Design review of the part built by this model. Coordinates are the model's own, in mm. Face numbers are marked on the shaded views. A direction names the side the tool comes from. Coordinates: 2 decimals unless noted, no trailing zeros. Write each loop counter-clockwise with the first axis right and the second up, starting at its lowest first coordinate (ties: lowest second). Pieces come first, ordered by that corner, then holes.
Q1. Take a section at B-B, the plane x = -13.5. Write out the cut boundary in (y, z), plus the area to 3 significant figures.
Q2. Take a section at C-C, the plane z = 41. Write out the cut boundary in (x, y), plus the area to 3 significant figures.
Q3. For the marked faces 1 and 2, list the 3-axis set-ups (+Z, -Z, +X, -X, +Y, -Y) from which the entire face can be reached by the end or side of a thin tool; tool diameter is ignored.
Q4. Take a section at A-A, the plane z = 52. Write out the cut boundary in (x, y), plus the area to 3 significant figures.
Q5. Take a section at D-D, the plane x = -29. Write out the cut boundary in (y, z).
Q6. For L1, parallel to Z at x = -37.5, y = 0.35; L2, parallel to Z at x = -13.5, y = 0.3; L3, parallel to Z at x = -11, y = 1.95, list the stretches that pass through material, from the lowest coordinate up.
Q7. For pin 1 Ø0.9 at (y, z) = (-0.5, 7.5) entering from -X; pin 2 Ø3.5 at (x, z) = (-37.5, 52) entering from +Y; pin 3 Ø0.7 at (x, y) = (-2, 0.5) entering from -Z, all flat-tipped, find the tip position at first contact; note any pin that passes through.
Autodesk Inventor part; units mm, degrees
ref_plane "YZ Plane" through (0, 0, 0) normal (1, 0, 0) x (0, 1, 0)
ref_plane "XZ Plane" through (0, 0, 0) normal (0, 1, 0) x (-1, 0, 0)
ref_plane "XY Plane" through (0, 0, 0) normal (0, 0, 1) x (1, 0, 0)
sketch "Sketch1" plane through (0, 0, 0) normal (0, 1, 0) x (-1, 0, 0)
  line L0 (40, 70) -> (0, 70)
  line L1 (0, 70) -> (0, 0)
  line L2 (0, 0) -> (40, 0)
  line L3 (40, 0) -> (40, 70)
  line L4 (0, 4) -> (7.5, 4)
  line L5 (7.5, 4) -> (7.5, 0)
  line L6 (7.5, 0) -> (0, 0)
  line L7 (0, 0) -> (0, 4)
  line L8 (0, 70) -> (7.5, 70)
  line L9 (7.5, 70) -> (7.5, 66)
  line L10 (7.5, 66) -> (0, 66)
  line L11 (0, 66) -> (0, 70)
  line L12 (0, 11) -> (3.0528, 11)
  line L13 (3.5, 11.4472) -> (3.5, 11.8944)
  line L14 (3.0528, 11.8944) -> (0, 11.8944)
  line L15 (0, 11.8944) -> (0, 11)
  arc A0 (3.0528, 11) -> (3.0528, 11.8944) centre (3.0528, 11.4472) ccw
  circle A1 centre (13.5, 3) radius 1.5
  circle A2 centre (13.5, 67) radius 1.5
  circle A3 centre (37.5, 52) radius 1.5
  circle A4 centre (37.5, 18) radius 1.5
  dimension "d0" = 70
  dimension "d1" = 40
  dimension "d2" = 0
  dimension "d3" = 0
  dimension "d4" = 7.5
  dimension "d5" = 7.5
  dimension "d6" = 4
  dimension "d7" = 4
  dimension "d8" = 1
  dimension "d9" = 11
  dimension "d10" = 3.5
  dimension "d13" = 3
  dimension "d14" = 3
  dimension "d15" = 3
  dimension "d16" = 3
  dimension "d17" = 13.5
  dimension "d18" = 13.5
  dimension "d19" = 3
  dimension "d20" = 3
  dimension "d21" = 2.5
  dimension "d22" = 2.5
  dimension "d23" = 18
  dimension "d24" = 18
extrude "Extrusion1" add sketch "Sketch1" along normal blind 1.4 contours L3 L2 L5 L4 L1 L12 A0 L14 L10 L9 L0
sketch "Sketch2" plane through (0, 1.4, 0) normal (0, 1, 0) x (1, 0, 0)
  line L0 (-30.8932, -46.4853) -> (-9.8932, -46.4853)
  line L1 (-9.8932, -46.4853) -> (-9.8932, -25.4853)
  line L2 (-9.8932, -25.4853) -> (-30.8932, -25.4853)
  line L3 (-30.8932, -25.4853) -> (-30.8932, -46.4853)
  point P0 (0, 0)
  dimension "d25" = 21
  dimension "d26" = 21
extrude "Extrusion2" add sketch "Sketch2" along normal blind 2.2
sketch "Sketch3" plane through (0, 1.4, 0) normal (0, 1, 0) x (1, 0, 0)
  line L0 (-35.3745, -15.5245) -> (-27.8702, -15.5245)
  line L1 (-27.8702, -15.5245) -> (-27.8702, -0.887)
  line L2 (-27.8702, -0.887) -> (-35.3745, -0.887)
  line L3 (-35.3745, -0.887) -> (-35.3745, -15.5245)
  line L4 (-24.8422, -15.5245) -> (-17.338, -15.5245)
  line L5 (-17.338, -15.5245) -> (-17.338, -0.887)
  line L6 (-17.338, -0.887) -> (-24.8422, -0.887)
  line L7 (-24.8422, -0.887) -> (-24.8422, -15.5245)
  point P0 (0, 0)
extrude "Extrusion3" add sketch "Sketch3" along normal blind 1.1 and the other way blind 2.5
sketch "Sketch4" plane through (0, 1.4, 0) normal (0, 1, 0) x (1, 0, 0)
  line L0 (-32.614, -64.2463) -> (-25.5454, -64.2463)
  line L1 (-25.5454, -64.2463) -> (-25.5454, -56.7849)
  line L2 (-25.5454, -56.7849) -> (-32.614, -56.7849)
  line L3 (-32.614, -56.7849) -> (-32.614, -64.2463)
  point P0 (0, 0)
extrude "Extrusion4" add sketch "Sketch4" along normal blind 1.1
sketch "Sketch5" plane through (0, 0, 0) normal (0, -1, 0) x (1, 0, 0)
  line L0 (-38.6782, 35.593) -> (-32.0822, 35.593)
  line L1 (-32.0822, 35.593) -> (-32.0822, 48.5473)
  line L2 (-32.0822, 48.5473) -> (-38.6782, 48.5473)
  line L3 (-38.6782, 48.5473) -> (-38.6782, 35.593)
  point P0 (0, 0)
extrude "Extrusion5" add sketch "Sketch5" along normal blind 1.1
properties part number "μQ7-962_Module"
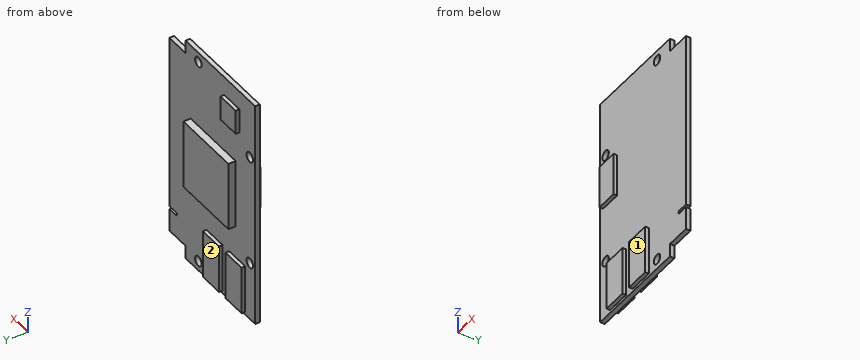
Responses:
1. outline: (0, 0) - (1.4, 0) - (1.4, 1.5) - (0, 1.5) - close; (0, 4.5) - (1.4, 4.5) - (1.4, 25.49) - (3.6, 25.49) - (3.6, 46.49) - (1.4, 46.49) - (1.4, 65.5) - (0, 65.5) - close; (0, 68.5) - (1.4, 68.5) - (1.4, 70) - (0, 70) - close
1. area: 136 mm2
2. outline: (-40, 0) - (-38.68, 0) - (-38.68, -1.1) - (-32.08, -1.1) - (-32.08, 0) - (0, 0) - (0, 1.4) - (-9.89, 1.4) - (-9.89, 3.6) - (-30.89, 3.6) - (-30.89, 1.4) - (-40, 1.4) - close
2. area: 109 mm2
3. face 1: +Z, -Z, +X, -X, -Y
3. face 2: -Z, +X, -X, +Y
4. outline: (-40, 0) - (-39, 0) - (-39, 1.4) - (-40, 1.4) - close; (-36, 0) - (0, 0) - (0, 1.4) - (-36, 1.4) - close
4. area: 51.8 mm2
5. outline: (-1.1, 0.89) - (0, 0.89) - (0, 0) - (1.4, 0) - (1.4, 0.89) - (2.5, 0.89) - (2.5, 15.52) - (1.4, 15.52) - (1.4, 25.49) - (3.6, 25.49) - (3.6, 46.49) - (1.4, 46.49) - (1.4, 56.78) - (2.5, 56.78) - (2.5, 64.25) - (1.4, 64.25) - (1.4, 70) - (0, 70) - (0, 15.52) - (-1.1, 15.52) - close
6. L1: z = 0 to 16.5, 19.5 to 50.5, 53.5 to 70
6. L2: z = 0 to 1.5, 4.5 to 65.5, 68.5 to 70
6. L3: z = 25.49 to 46.49
7. pin 1: stops at x = -35.37
7. pin 2: stops at y = 1.4
7. pin 3: stops at z = 4
